The listing builds one solid part. Answer for the finished solid, in the listing's coordinates (mm). A direction names the side the tool comes from. Coordinates: 2 decimals unless noted, no trailing zeros. Loops run counter-clockwise (first coordinate to the right, second up) from the corner with the lowest first, then second, coordinate; pieces in that order, holes last. Notation, with made-up numbers: M 18,48 L 52,48 A24 cw 52,61 Z; hole C 37,40.25 d11. An arc over 180 degrees is marked long. Answer as a JSON object with one key per item and string values. Group by question number.
1. A cutting plane is placed at A-A on y = 50.5. Give the vertices of the cut face in (x, z).
2. Straight lines are drawn through the part: L1, parallel to X at y = 6, z = -0.5; L2, parallel to Z at x = 0, y = 7; L3, parallel to Y at x = 1.5, z = -26. For each, find the intervals that lie inside material, in ascending order.
3. Given pin 1 (11 mm diameter, centred on x = 28, y = 82.5, fed in from -Z); pin 2 (2 mm diameter, centred on x = -31, z = 4.5, fed in from -Y); pin 3 (5 mm diameter, centred on y = 73, z = 5.5, fed in from -X), each flat-ended and moving along its own axis, determine where each tip first touches the part or whether it passes through.
4. A cutting plane is placed at B-B on x = 0. Give the vertices of the cut face in (y, z).
5. Determine the mould class of faces 1 (the face through (24, 109, 0)), 2 (the face through (-31.3, 107, -0.1)), 3 (the face through (26, 64, 10)) for opening direction Z: released by +Z, released by -Z, zero draft, split by the parting line, or undercut.
6. For faces 4 (the face through (25.14, 105, -0.79)), 5 (the face through (-24, 109, 0)), 6 (the face through (31.2, 107, -0.1)), 7 (the face through (0.1, 30, -28.7)), determine the directions among +Z, -Z, +X, -X, +Y, -Y from which every point of the face is accessible in a straight line to the end or side of a thin tool.
from build123d import *

# Parameters (mm, degrees)
SKETCH1_R           = 29
SKETCH1_R_2         = 27
BOSS_EXTRUDE1_DEPTH = 30
BOSS_EXTRUDE2_START = 2
SKETCH2_R           = 29
BOSS_EXTRUDE2_DEPTH = 2
BOSS_EXTRUDE3_DEPTH = 75
BOSS_EXTRUDE5_DEPTH = 2
FILLET2_R           = 1
BOSS_EXTRUDE6_DEPTH = 5
FILLET3_R           = 2
SKETCH7_W           = 70
SKETCH7_H           = 116
CUT_EXTRUDE1_DEPTH  = 19


with BuildPart() as part:
    # Sketch1 → Boss-Extrude1 (new body)
    with BuildSketch(Plane(origin=(0, 0, 0), x_dir=(1, 0, 0), z_dir=(0, 1, 0))):
        with Locations(Location((0, 0, 0), (0, 0, 270))):
            Circle(SKETCH1_R)
        with Locations(Location((0, 0, 0), (0, 0, 270))):
            Circle(SKETCH1_R_2, mode=Mode.SUBTRACT)
    extrude(amount=BOSS_EXTRUDE1_DEPTH)

    # Sketch2 → Boss-Extrude2 (add)
    with BuildSketch(Plane.XZ.offset(BOSS_EXTRUDE2_START)):
        with Locations(Location((0, 0, 0), (0, 0, 270))):
            Circle(SKETCH2_R)
    extrude(amount=-BOSS_EXTRUDE2_DEPTH)

    # Sketch3 → Boss-Extrude3 (add)
    with BuildSketch(Plane(origin=(0, 30, 0), x_dir=(1, 0, 0), z_dir=(0, 1, 0))):
        with BuildLine():
            ThreePointArc((27.221315178, -10), (29, 0), (27.221315178, 10))
            Line((27.221315178, 10), (25.079872408, 10))
            ThreePointArc((25.079872408, 10), (27, 0), (25.079872408, -10))
            Line((25.079872408, -10), (27.221315178, -10))
        make_face()
        with BuildLine():
            Line((-25.079872408, 10), (-27.221315178, 10))
            ThreePointArc((-27.221315178, 10), (-29, 0), (-27.221315178, -10))
            Line((-27.221315178, -10), (-25.079872408, -10))
            ThreePointArc((-25.079872408, -10), (-27, 0), (-25.079872408, 10))
        make_face()
    extrude(amount=BOSS_EXTRUDE3_DEPTH)

    # Sketch4 → Boss-Extrude5 (add)
    with BuildSketch(Plane(origin=(0, 105, 0), x_dir=(1, 0, 0), z_dir=(0, 1, 0))):
        with BuildLine():
            ThreePointArc((25.079872408, -10), (27, 0), (25.079872408, 10))
            Line((25.079872408, 10), (21.817424229, 10))
            ThreePointArc((21.817424229, 10), (23.448008247, 5.117705467), (24, 0))
            ThreePointArc((24, 0), (23.448008247, -5.117705467), (21.817424229, -10))
            Line((21.817424229, -10), (25.079872408, -10))
        make_face()
        with BuildLine():
            ThreePointArc((25.079872408, 10), (27, 0), (25.079872408, -10))
            Line((25.079872408, -10), (27.221315178, -10))
            ThreePointArc((27.221315178, -10), (29, 0), (27.221315178, 10))
            Line((27.221315178, 10), (25.079872408, 10))
        make_face()
        with BuildLine():
            Line((-21.817424229, 10), (-27.221315178, 10))
            ThreePointArc((-27.221315178, 10), (-28.551866312, 5.078477145), (-29, 3.9e-08))
            ThreePointArc((-29, 3.9e-08), (-28.551866318, -5.078477108), (-27.221315178, -10))
            Line((-27.221315178, -10), (-21.817424229, -10))
            ThreePointArc((-21.817424229, -10), (-24, 0), (-21.817424229, 10))
        make_face()
    extrude(amount=BOSS_EXTRUDE5_DEPTH)

    # Fillet2
    # the kernel refuses this fillet: 1 mm, written as the material it adds along each edge
    with BuildSketch(Plane(origin=(0, 105, 0), x_dir=(0.8906566474761322, 0, -0.4546765183144792), z_dir=(-0.4546765183144792, 0, -0.8906566474761322))) as fillet2_piece_1_section:
        with BuildLine():
            CenterArc((27 - FILLET2_R, FILLET2_R), FILLET2_R, 270, 90)
            Line((27 - FILLET2_R, 0), (27, 0))
            Line((27, 0), (27, FILLET2_R))
        make_face()
    fillet2_piece_1 = revolve(axis=Axis((0, 105, 0), (0, -1, 0)), revolution_arc=54.088245562, mode=Mode.PRIVATE)
    fillet2_piece_1 = split(fillet2_piece_1, bisect_by=Plane(origin=(26.719378233, 104.719378233, 10), z_dir=(0, 0, -1)), keep=Keep.TOP, mode=Mode.PRIVATE)
    fillet2_piece_1 = split(fillet2_piece_1, bisect_by=Plane(origin=(26.719378233, 104.719378233, -10), z_dir=(0, 0, 1)), keep=Keep.TOP, mode=Mode.PRIVATE)
    add(fillet2_piece_1)
    with BuildSketch(Plane(origin=(0, 105, 0), x_dir=(-0.890656647476122, 0, 0.4546765183144991), z_dir=(0.4546765183144991, 0, 0.890656647476122))) as fillet2_piece_2_section:
        with BuildLine():
            CenterArc((27 - FILLET2_R, FILLET2_R), FILLET2_R, 270, 90)
            Line((27 - FILLET2_R, 0), (27, 0))
            Line((27, 0), (27, FILLET2_R))
        make_face()
    fillet2_piece_2 = revolve(axis=Axis((0, 105, 0), (0, -1, 0)), revolution_arc=54.088245562, mode=Mode.PRIVATE)
    fillet2_piece_2 = split(fillet2_piece_2, bisect_by=Plane(origin=(-26.719378233, 104.719378233, 10), z_dir=(0, 0, -1)), keep=Keep.TOP, mode=Mode.PRIVATE)
    fillet2_piece_2 = split(fillet2_piece_2, bisect_by=Plane(origin=(-26.719378233, 104.719378233, -10), z_dir=(0, 0, 1)), keep=Keep.TOP, mode=Mode.PRIVATE)
    add(fillet2_piece_2)
    with BuildSketch(Plane(origin=(0, 0, 0), x_dir=(0, 0, 1), z_dir=(-1, 0, 0))) as fillet2_piece_3:
        with BuildLine():
            CenterArc((27 - FILLET2_R, FILLET2_R), FILLET2_R, 270, 90)
            Line((27 - FILLET2_R, 0), (27, 0))
            Line((27, 0), (27, FILLET2_R))
        make_face()
    revolve(axis=Axis((0, 0, 0), (0, 1, 0)))
    # the kernel refuses this fillet: 1 mm, written as the material it takes off along each edge
    with BuildSketch(Plane(origin=(0, 30, 0), x_dir=(0.9591739549871109, 0, -0.28281676766836794), z_dir=(0.28281676766836794, 0, 0.9591739549871109))) as fillet2_2_piece_1_section:
        with BuildLine():
            CenterArc((27 + FILLET2_R, -FILLET2_R), FILLET2_R, 90, 90)
            Line((27, -FILLET2_R), (27, 0))
            Line((27, 0), (27 + FILLET2_R, 0))
        make_face()
    fillet2_2_piece_1 = revolve(axis=Axis((0, 30, 0), (0, 1, 0)), revolution_arc=147.143219234, mode=Mode.PRIVATE)
    fillet2_2_piece_1 = split(fillet2_2_piece_1, bisect_by=Plane(origin=(0, 29.725140897, -10), z_dir=(0, 0, -1)), keep=Keep.TOP, mode=Mode.PRIVATE)
    add(fillet2_2_piece_1, mode=Mode.SUBTRACT)
    with BuildSketch(Plane(origin=(0, 30, 0), x_dir=(-0.9591557890892681, 0, 0.28287837007545047), z_dir=(-0.28287837007545047, 0, -0.9591557890892681))) as fillet2_2_piece_2_section:
        with BuildLine():
            CenterArc((27 + FILLET2_R, -FILLET2_R), FILLET2_R, 90, 90)
            Line((27, -FILLET2_R), (27, 0))
            Line((27, 0), (27 + FILLET2_R, 0))
        make_face()
    fillet2_2_piece_2 = revolve(axis=Axis((0, 30, 0), (0, 1, 0)), revolution_arc=73.567929793, mode=Mode.PRIVATE)
    fillet2_2_piece_2 = split(fillet2_2_piece_2, bisect_by=Plane(origin=(-15.465500951, 29.721420389, 10), z_dir=(0, 0, 1)), keep=Keep.TOP, mode=Mode.PRIVATE)
    add(fillet2_2_piece_2, mode=Mode.SUBTRACT)
    with BuildSketch(Plane(origin=(0, 105, 0), x_dir=(0.8608011340646036, 0, -0.5089414579232981), z_dir=(-0.5089414579232981, 0, -0.8608011340646036))) as fillet2_2_piece_3:
        with BuildLine():
            CenterArc((24 + FILLET2_R, -FILLET2_R), FILLET2_R, 90, 90)
            Line((24 + FILLET2_R, 0), (24, 0))
            Line((24, 0), (24, -FILLET2_R))
        make_face()
    revolve(axis=Axis((0, 105, 0), (0, -1, 0)), revolution_arc=61.186692958, mode=Mode.SUBTRACT)
    with BuildSketch(Plane(origin=(0, 105, 0), x_dir=(-0.860801134064602, 0, 0.5089414579233009), z_dir=(0.5089414579233009, 0, 0.860801134064602))) as fillet2_2_piece_4:
        with BuildLine():
            CenterArc((24 + FILLET2_R, -FILLET2_R), FILLET2_R, 90, 90)
            Line((24 + FILLET2_R, 0), (24, 0))
            Line((24, 0), (24, -FILLET2_R))
        make_face()
    revolve(axis=Axis((0, 105, 0), (0, -1, 0)), revolution_arc=61.186692958, mode=Mode.SUBTRACT)
    with BuildSketch(Plane(origin=(0, 30, 0), x_dir=(0, 0, 1), z_dir=(-1, 0, 0))) as fillet2_2_piece_5_section:
        with BuildLine():
            CenterArc((27 + FILLET2_R, -FILLET2_R), FILLET2_R, 90, 90)
            Line((27, -FILLET2_R), (27, 0))
            Line((27, 0), (27 + FILLET2_R, 0))
        make_face()
    fillet2_2_piece_5 = revolve(axis=Axis((0, 30, 0), (0, 1, 0)), revolution_arc=73.567929793, mode=Mode.PRIVATE)
    fillet2_2_piece_5 = split(fillet2_2_piece_5, bisect_by=Plane(origin=(15.465500935, 29.721420416, 10), z_dir=(0, 0, 1)), keep=Keep.TOP, mode=Mode.PRIVATE)
    add(fillet2_2_piece_5, mode=Mode.SUBTRACT)

    # Sketch6 → Boss-Extrude6 (add)
    with BuildSketch(Plane(origin=(0, 107, 0), x_dir=(1, 0, 0), z_dir=(0, 1, 0))):
        with BuildLine():
            ThreePointArc((-27.221315178, -10), (-29, 0), (-27.221315178, 10))
            Line((-27.221315178, 10), (-34, 10))
            Line((-34, 10), (-34, -10))
            Line((-34, -10), (-27.221315178, -10))
        make_face()
        with BuildLine():
            Line((-27.221315178, -10), (-21.817424229, -10))
            ThreePointArc((-21.817424229, -10), (-24, 0), (-21.817424229, 10))
            Line((-21.817424229, 10), (-27.221315178, 10))
            ThreePointArc((-27.221315178, 10), (-29, 0), (-27.221315178, -10))
        make_face()
        with BuildLine():
            Line((34, 10), (21.817424229, 10))
            ThreePointArc((21.817424229, 10), (23.448008247, 5.117705467), (24, 0))
            ThreePointArc((24, 0), (23.448008247, -5.117705467), (21.817424229, -10))
            Line((21.817424229, -10), (34, -10))
            Line((34, -10), (34, 10))
        make_face()
    extrude(amount=BOSS_EXTRUDE6_DEPTH)

    # Fillet3
    # the kernel refuses this fillet: 2 mm, written as the material it adds along each edge
    with BuildSketch(Plane(origin=(0, 107, 0), x_dir=(0.8655830504384638, 0, 0.5007653969611356), z_dir=(-0.5007653969611356, 0, 0.8655830504384638))) as fillet3_piece_1_section:
        with BuildLine():
            CenterArc((29 + FILLET3_R, -FILLET3_R), FILLET3_R, 90, 90)
            Line((29 + FILLET3_R, 0), (29, 0))
            Line((29, 0), (29, -FILLET3_R))
        make_face()
    fillet3_piece_1 = revolve(axis=Axis((0, 107, 0), (0, 1, 0)), revolution_arc=60.101302376, mode=Mode.PRIVATE)
    fillet3_piece_1 = split(fillet3_piece_1, bisect_by=Plane(origin=(29.566335582, 106.433664418, -10), z_dir=(0, 0, 1)), keep=Keep.TOP, mode=Mode.PRIVATE)
    fillet3_piece_1 = split(fillet3_piece_1, bisect_by=Plane(origin=(29.566335582, 106.433664418, 10), z_dir=(0, 0, -1)), keep=Keep.TOP, mode=Mode.PRIVATE)
    add(fillet3_piece_1)
    with BuildSketch(Plane(origin=(0, 107, 0), x_dir=(-0.8655830504384671, 0, 0.5007653969611302), z_dir=(0.5007653969611302, 0, 0.8655830504384671))) as fillet3_piece_2_section:
        with BuildLine():
            CenterArc((29 + FILLET3_R, FILLET3_R), FILLET3_R, 180, 90)
            Line((29 + FILLET3_R, 0), (29, 0))
            Line((29, 0), (29, FILLET3_R))
        make_face()
    fillet3_piece_2 = revolve(axis=Axis((0, 107, 0), (0, -1, 0)), revolution_arc=60.101302376, mode=Mode.PRIVATE)
    fillet3_piece_2 = split(fillet3_piece_2, bisect_by=Plane(origin=(-29.566335582, 106.433664418, 10), z_dir=(0, 0, -1)), keep=Keep.TOP, mode=Mode.PRIVATE)
    fillet3_piece_2 = split(fillet3_piece_2, bisect_by=Plane(origin=(-29.566335582, 106.433664418, -10), z_dir=(0, 0, 1)), keep=Keep.TOP, mode=Mode.PRIVATE)
    add(fillet3_piece_2)
    # the kernel refuses this fillet: 2 mm, written as the material it takes off along each edge
    with BuildSketch(Plane(origin=(-34, 107, -15), x_dir=(0, 1, 0), z_dir=(0, 0, 1)), Plane(origin=(34, 107, 15), x_dir=(0, 1, 0), z_dir=(0, 0, -1))) as fillet3_2_piece_1:
        with BuildLine():
            CenterArc((FILLET3_R, -FILLET3_R), FILLET3_R, 90, 90)
            Line((0, -FILLET3_R), (0, 0))
            Line((0, 0), (FILLET3_R, 0))
        make_face()
    extrude(amount=30, mode=Mode.SUBTRACT)
    with BuildSketch(Plane(origin=(-34, 102, -10), x_dir=(0, 0, 1), z_dir=(0, 1, 0)), Plane(origin=(-34, 102, 10), x_dir=(1, 0, 0), z_dir=(0, 1, 0)), Plane(origin=(34, 102, 10), x_dir=(0, 0, -1), z_dir=(0, 1, 0)), Plane(origin=(34, 102, -10), x_dir=(-1, 0, 0), z_dir=(0, 1, 0))) as fillet3_2_piece_2:
        with BuildLine():
            CenterArc((FILLET3_R, FILLET3_R), FILLET3_R, 180, 90)
            Line((0, FILLET3_R), (0, 0))
            Line((0, 0), (FILLET3_R, 0))
        make_face()
    extrude(amount=15, mode=Mode.SUBTRACT)
    with BuildSketch(Plane(origin=(-34, 112, -15), x_dir=(0, -1, 0), z_dir=(0, 0, 1)), Plane(origin=(34, 112, 15), x_dir=(0, -1, 0), z_dir=(0, 0, -1))) as fillet3_2_piece_3:
        with BuildLine():
            CenterArc((FILLET3_R, FILLET3_R), FILLET3_R, 180, 90)
            Line((0, FILLET3_R), (0, 0))
            Line((0, 0), (FILLET3_R, 0))
        make_face()
    extrude(amount=30, mode=Mode.SUBTRACT)

    # Sketch7 → Cut-Extrude1 (cut)
    with BuildSketch(Plane.XY.offset(29)):
        with Locations((0, 55)):
            Rectangle(SKETCH7_W, SKETCH7_H)
    extrude(amount=-CUT_EXTRUDE1_DEPTH, mode=Mode.SUBTRACT)


solid = part.part
From the geometry:
{
 "1": {"outline": "M -27.22,-10 L -25.08,-10 A27 cw -25.08,10 L -27.22,10 A29 ccw Z; M 25.08,-10 L 27.22,-10 A29 ccw 27.22,10 L 25.08,10 A27 cw Z"},
 "2": {"L1": "x = -29 to -27, 27 to 29", "L2": "z = -29 to -27", "L3": "y = -2 to 0"},
 "3": {"pin 1": "stops at z = -10", "pin 2": "stops at y = 106.88", "pin 3": "stops at x = -28.84"},
 "4": {"outline": "M -2,-29 L 30,-29 L 30,-28 A1 ccw 29,-27 L 1,-27 A1 cw 0,-26 L 0,10 L -2,10 Z"},
 "5": {"face 1": "undercut", "face 2": "zero draft", "face 3": "released by +Z"},
 "6": {"face 4": "none", "face 5": "+Y", "face 6": "+X, -Y", "face 7": "-Z, +X, -X, +Y"}
}
